```python
from build123d import *

# Parameters (mm, degrees)
F1_DEPTH = 15
F3_DEPTH = 25
F4_R     = 2
F5_DEPTH = 15


with BuildPart() as f1:
    # F0 (on Front) → F1 (new body)
    with BuildSketch(Plane.XZ):
        Polygon((1.792286, 40.719454), (-2.707714, 40.719454), (-2.707714, -9.280546), (12.292286, -9.280546), (12.292286, 40.719454), (7.792286, 40.719454), (4.792286, 37.719454), align=None)
    extrude(amount=F1_DEPTH)

    # F2 (on face) → F3 (cut)
    with BuildSketch(Plane.YZ.offset(12.292286)):
        Polygon((-15, 3.398946), (-5, 40.719454), (-15, 40.719454), align=None)
    extrude(amount=-F3_DEPTH, mode=Mode.SUBTRACT)

    # F4 (on face) → F5 (cut)
    with BuildSketch(Plane(origin=(0, 0, -9.280546), x_dir=(1, 0, 0), z_dir=(0, 0, -1))):
        with Locations((4.792286, 7.5)):
            Circle(F4_R)
    extrude(amount=-F5_DEPTH, mode=Mode.SUBTRACT)


solid = f1.part
```
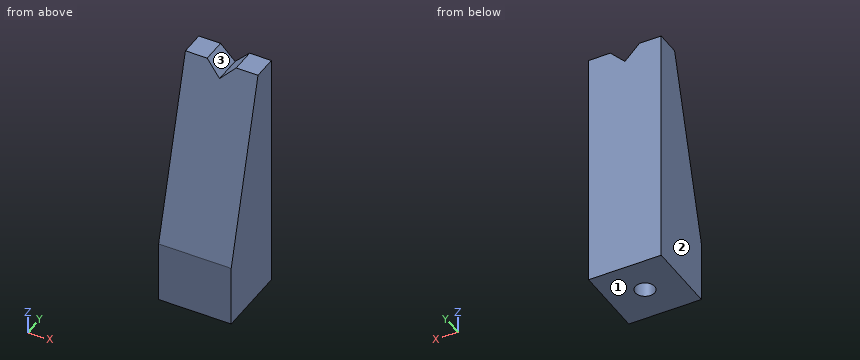
Build history of the part. All positions in model axes, mm. Face numbers are marked on the shaded views. Coordinates: 2 decimals unless noted, no trailing zeros. Order: outer loops, then holes, each group sorted by start corner. A loop starts at its lowest first (then second) coordinate and runs counter-clockwise, first axis right, second up.
Item 1: Drill centre lines: L1, parallel to X at y = -7.5, z = 1.75; L2, parallel to Y at x = 5.5, z = 2; L3, parallel to Z at x = 4.75, y = -3.75. Where is each one in solid material? Low to high.
Filled in:
L1: x = -2.71 to 2.79, 6.79 to 12.29
L2: y = -15 to -9.37, -5.63 to 0
L3: z = -9.28 to 37.76
Item 2: Drop flat-ended pins along their axis: pin 1 Ø2 at (x, z) = (8, 21) entering from -Y; pin 2 Ø1.2 at (x, y) = (4, -7.5) entering from -Z. Give the stop position or say it passes through.
Filled in:
pin 1: stops at y = -10.55
pin 2: stops at z = 5.72
Item 3: Saw through at B-B on z = 16.5. List the corners of the cut face in (x, y), then the cut area to 3 significant figures.
Filled in:
outline: (-2.71, -11.49) - (12.29, -11.49) - (12.29, 0) - (-2.71, 0) - close
area: 172 mm2
Item 4: Saw through at C-C on z = 37. List the corners of the cut face in (x, y), then the cut area to 3 significant figures.
Filled in:
outline: (-2.71, -6) - (12.29, -6) - (12.29, 0) - (-2.71, 0) - close
area: 89.9 mm2
Item 5: Saw through at A-A on y = -7.5. List the corners of the cut face in (x, z), then the cut area to 3 significant figures.
Filled in:
outline: (-2.71, -9.28) - (2.79, -9.28) - (2.79, 5.72) - (6.79, 5.72) - (6.79, -9.28) - (12.29, -9.28) - (12.29, 31.39) - (-2.71, 31.39) - close
area: 550 mm2
Item 6: Mould opens along X. For the marked faces 1, 2 and 3 say: released by +X, released by -X, zero draft, split by the parting line, or undercut.
Filled in:
face 1: zero draft
face 2: released by -X
face 3: undercut
